from build123d import *

# Parameters (mm, degrees)
SKETCH1_W                                      = 250
SKETCH1_H                                      = 95
SKETCH1_W_2                                    = 230
SKETCH1_H_2                                    = 75
BOSS_EXTRUDE1_DEPTH                            = 15
FILLET1_R                                      = 3
CUT_EXTRUDE2_DEPTH                             = 16
CBORE_FOR_M1_6_HEX_HEAD_CAP_SCREW1_D           = 3
CBORE_FOR_M1_6_HEX_HEAD_CAP_SCREW1_CBORE_D     = 5
CBORE_FOR_M1_6_HEX_HEAD_CAP_SCREW1_CBORE_DEPTH = 5


with BuildPart() as part:
    # Sketch1 → Boss-Extrude1 (new body)
    with BuildSketch(Plane.XY):
        with Locations((125, 47.5)):
            Rectangle(SKETCH1_W, SKETCH1_H)
        with Locations((125, 47.5)):
            Rectangle(SKETCH1_W_2, SKETCH1_H_2, mode=Mode.SUBTRACT)
        Polygon((40, 85), (10, 63), (10, 56.799641587), (48.455034199, 85), align=None)
        Polygon((48.455034199, 10), (10, 38.200358413), (10, 32), (40, 10), align=None)
        Polygon((240, 38.200358413), (201.544965801, 10), (210, 10), (240, 32), align=None)
        Polygon((210, 85), (201.544965801, 85), (240, 56.799641587), (240, 63), align=None)
    extrude(amount=BOSS_EXTRUDE1_DEPTH)

    # Fillet1
    fillet1_edges = [part.edges().sort_by_distance(p)[0] for p in [
        (10, 32, 7.5),
        (10, 10, 7.5),
        (40, 10, 7.5),
        (210, 10, 7.5),
        (240, 10, 7.5),
        (240, 32, 7.5),
        (240, 63, 7.5),
        (240, 85, 7.5),
        (210, 85, 7.5),
        (10, 85, 7.5),
        (10, 63, 7.5),
        (40, 85, 7.5),
        (48.455034199, 85, 7.5),
        (10, 56.799641587, 7.5),
        (10, 38.200358413, 7.5),
        (48.455034199, 10, 7.5),
        (201.544965801, 10, 7.5),
        (240, 38.200358413, 7.5),
        (240, 56.799641587, 7.5),
        (201.544965801, 85, 7.5),
    ]]
    fillet(fillet1_edges, radius=FILLET1_R)

    # Sketch11 → Cut-Extrude2 (cut, through all)
    with BuildSketch(Plane(origin=(0, 0, 0), x_dir=(-1, 0, 0), z_dir=(0, 0, -1))):
        with BuildLine():
            Line((-248, 80), (-248, 55))
            ThreePointArc((-248, 55), (-245, 52), (-242, 55))
            Line((-242, 55), (-242, 80))
            ThreePointArc((-242, 80), (-245, 83), (-248, 80))
        make_face()
        with BuildLine():
            Line((-248, 40), (-248, 15))
            ThreePointArc((-248, 15), (-245, 12), (-242, 15))
            Line((-242, 15), (-242, 40))
            ThreePointArc((-242, 40), (-245, 43), (-248, 40))
        make_face()
        with BuildLine():
            Line((-190, 8), (-235, 8))
            ThreePointArc((-235, 8), (-238, 5), (-235, 2))
            Line((-235, 2), (-190, 2))
            ThreePointArc((-190, 2), (-187, 5), (-190, 8))
        make_face()
        with BuildLine():
            Line((-130, 8), (-180, 8))
            ThreePointArc((-180, 8), (-183, 5), (-180, 2))
            Line((-180, 2), (-130, 2))
            ThreePointArc((-130, 2), (-127, 5), (-130, 8))
        make_face()
        with BuildLine():
            Line((-70, 8), (-120, 8))
            ThreePointArc((-120, 8), (-123, 5), (-120, 2))
            Line((-120, 2), (-70, 2))
            ThreePointArc((-70, 2), (-67, 5), (-70, 8))
        make_face()
        with BuildLine():
            Line((-15, 8), (-60, 8))
            ThreePointArc((-60, 8), (-63, 5), (-60, 2))
            Line((-60, 2), (-15, 2))
            ThreePointArc((-15, 2), (-12, 5), (-15, 8))
        make_face()
        with BuildLine():
            Line((-8, 40), (-8, 15))
            ThreePointArc((-8, 15), (-5, 12), (-2, 15))
            Line((-2, 15), (-2, 40))
            ThreePointArc((-2, 40), (-5, 43), (-8, 40))
        make_face()
        with BuildLine():
            Line((-8, 80), (-8, 55))
            ThreePointArc((-8, 55), (-5, 52), (-2, 55))
            Line((-2, 55), (-2, 80))
            ThreePointArc((-2, 80), (-5, 83), (-8, 80))
        make_face()
        with BuildLine():
            Line((-15, 93), (-60, 93))
            ThreePointArc((-60, 93), (-63, 90), (-60, 87))
            Line((-60, 87), (-15, 87))
            ThreePointArc((-15, 87), (-12, 90), (-15, 93))
        make_face()
        with BuildLine():
            Line((-70, 93), (-120, 93))
            ThreePointArc((-120, 93), (-123, 90), (-120, 87))
            Line((-120, 87), (-70, 87))
            ThreePointArc((-70, 87), (-67, 90), (-70, 93))
        make_face()
        with BuildLine():
            Line((-130, 93), (-180, 93))
            ThreePointArc((-180, 93), (-183, 90), (-180, 87))
            Line((-180, 87), (-130, 87))
            ThreePointArc((-130, 87), (-127, 90), (-130, 93))
        make_face()
        with BuildLine():
            Line((-190, 93), (-235, 93))
            ThreePointArc((-235, 93), (-238, 90), (-235, 87))
            Line((-235, 87), (-190, 87))
            ThreePointArc((-190, 87), (-187, 90), (-190, 93))
        make_face()
    extrude(amount=-CUT_EXTRUDE2_DEPTH, mode=Mode.SUBTRACT)

    # CBORE for M1.6 Hex Head Cap Screw1 (through all)
    with Locations(Plane(origin=(0, 0, 0), x_dir=(-1, 0, 0), z_dir=(0, 0, -1))):
        with Locations((-245, 90), (-245, 5), (-5, 5), (-5, 90)):
            CounterBoreHole(CBORE_FOR_M1_6_HEX_HEAD_CAP_SCREW1_D / 2, CBORE_FOR_M1_6_HEX_HEAD_CAP_SCREW1_CBORE_D / 2, CBORE_FOR_M1_6_HEX_HEAD_CAP_SCREW1_CBORE_DEPTH)


solid = part.part
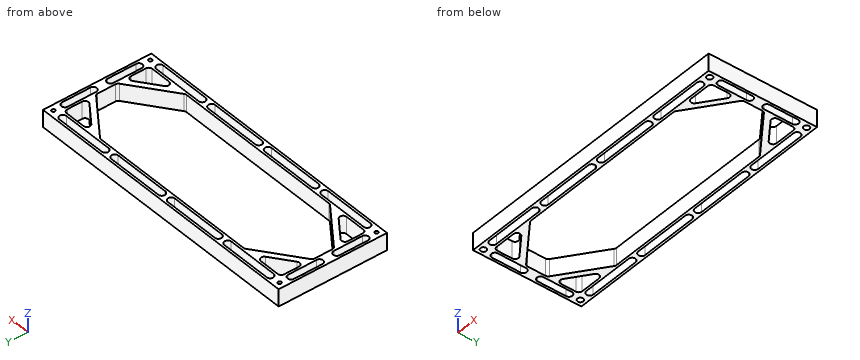
CAD build for the part. Positions are in the model's coordinates, mm. Round coordinates to 2 decimals unless told otherwise and drop trailing zeros. Write each loop counter-clockwise with the first axis right and the second up, starting at its lowest first coordinate (ties: lowest second). Pieces come first, ordered by that corner, then holes. Notation, with made-up numbers: M 24,36 L 50,36 A26 ccw 50,60 Z; hole C -6.5,39 d1. An arc over 180 degrees is marked long. Use a Markdown table: item, result. Add a question column.
1. Drill centre lines: probe 1 along Y at (x, z) = (139, 12); probe 2 along Y at (x, z) = (5, 1.9); probe 3 along X at (y, z) = (55.5, 3). Where is each one in solid material? Low to high.
2. Slice it at A-A on x = 113. Give the cut face in (y, z), then the cut area to 3 significant figures.
3. Flat gauge pin, fed straight in: P1, Ø4, axis at x = 245, y = 90, coming from the -Z side. Where does the tip first touch, or does it go through?
4. Slice it at B-B on z = 12.5. Give the number of separate pieces and of enclosed holes in the cut face, then the cut area to 3 significant figures.
5. Slice it at C-C on y = 18. Give the cut face in (x, z).
Reply:
| question | item | result |
|---|---|---|
| 1 | probe 1 | y = 0 to 2, 8 to 10, 85 to 87, 93 to 95 |
| 1 | probe 2 | y = 0 to 2.5, 7.5 to 12, 43 to 52, 83 to 87.5, 92.5 to 95 |
| 1 | probe 3 | x = 0 to 2, 8 to 10.01, 239.99 to 242, 248 to 250 |
| 2 | outline | M 0,0 L 2,0 L 2,15 L 0,15 Z; M 8,0 L 10,0 L 10,15 L 8,15 Z; M 85,0 L 87,0 L 87,15 L 85,15 Z; M 93,0 L 95,0 L 95,15 L 93,15 Z |
| 2 | area | 120 mm^2 |
| 3 | P1 | stops at z = 5 |
| 4 | separate pieces | 1 |
| 4 | enclosed holes | 21 |
| 4 | area | 4,210 mm^2 |
| 5 | outline | M 0,0 L 2,0 L 2,15 L 0,15 Z; M 8,0 L 10,0 L 10,15 L 8,15 Z; M 29.09,0 L 37.55,0 L 37.55,15 L 29.09,15 Z; M 212.45,0 L 220.91,0 L 220.91,15 L 212.45,15 Z; M 240,0 L 242,0 L 242,15 L 240,15 Z; M 248,0 L 250,0 L 250,15 L 248,15 Z |
